Check sheet for the modelled part. Datum: model origin and axes. Units: mm. Give positions to 0.01 mm unless a question says otherwise; leave off trailing zeros. Order: outer loops, then holes, each group sorted by start corner. A loop starts at its lowest first (then second) coordinate and runs counter-clockwise, first axis right, second up.
from build123d import *

# Parameters (mm, degrees)
SKETCH1_W           = 85
SKETCH1_H           = 155
BOSS_EXTRUDE1_DEPTH = 20
SKETCH3_R           = 5.05
CUT_EXTRUDE1_DEPTH  = 10
SKETCH5_W           = 15
SKETCH5_H           = 50
BOSS_EXTRUDE2_DEPTH = 5
SKETCH6_R           = 3
CUT_EXTRUDE2_DEPTH  = 5


with BuildPart() as part:
    # Sketch1 → Boss-Extrude1 (new body)
    with BuildSketch(Plane(origin=(0, 0, 0), x_dir=(1, 0, 0), z_dir=(0, 1, 0))):
        with Locations((42.5, 77.5)):
            Rectangle(SKETCH1_W, SKETCH1_H)
    extrude(amount=BOSS_EXTRUDE1_DEPTH)

    # Sketch3 → Cut-Extrude1 (cut)
    with BuildSketch(Plane(origin=(0, 20, 0), x_dir=(1, 0, 0), z_dir=(0, 1, 0))):
        with Locations(Location((10, 145, 0), (0, 0, 270))):
            Circle(SKETCH3_R)
        with Locations(Location((25, 145, 0), (0, 0, 270))):
            Circle(SKETCH3_R)
        with Locations(Location((40, 145, 0), (0, 0, 270))):
            Circle(SKETCH3_R)
        with Locations(Location((55, 145, 0), (0, 0, 270))):
            Circle(SKETCH3_R)
        with Locations(Location((70, 145, 0), (0, 0, 270))):
            Circle(SKETCH3_R)
        with Locations(Location((70, 130, 0), (0, 0, 270))):
            Circle(SKETCH3_R)
        with Locations(Location((55, 130, 0), (0, 0, 270))):
            Circle(SKETCH3_R)
        with Locations(Location((40, 130, 0), (0, 0, 270))):
            Circle(SKETCH3_R)
        with Locations(Location((25, 130, 0), (0, 0, 270))):
            Circle(SKETCH3_R)
        with Locations(Location((10, 130, 0), (0, 0, 270))):
            Circle(SKETCH3_R)
        with Locations(Location((70, 115, 0), (0, 0, 270))):
            Circle(SKETCH3_R)
        with Locations(Location((55, 115, 0), (0, 0, 270))):
            Circle(SKETCH3_R)
        with Locations(Location((40, 115, 0), (0, 0, 270))):
            Circle(SKETCH3_R)
        with Locations(Location((25, 115, 0), (0, 0, 270))):
            Circle(SKETCH3_R)
        with Locations(Location((10, 115, 0), (0, 0, 270))):
            Circle(SKETCH3_R)
        with Locations(Location((70, 100, 0), (0, 0, 270))):
            Circle(SKETCH3_R)
        with Locations(Location((55, 100, 0), (0, 0, 270))):
            Circle(SKETCH3_R)
        with Locations(Location((40, 100, 0), (0, 0, 270))):
            Circle(SKETCH3_R)
        with Locations(Location((25, 100, 0), (0, 0, 270))):
            Circle(SKETCH3_R)
        with Locations(Location((10, 100, 0), (0, 0, 270))):
            Circle(SKETCH3_R)
        with Locations(Location((70, 85, 0), (0, 0, 270))):
            Circle(SKETCH3_R)
        with Locations(Location((55, 85, 0), (0, 0, 270))):
            Circle(SKETCH3_R)
        with Locations(Location((40, 85, 0), (0, 0, 270))):
            Circle(SKETCH3_R)
        with Locations(Location((25, 85, 0), (0, 0, 270))):
            Circle(SKETCH3_R)
        with Locations(Location((10, 85, 0), (0, 0, 270))):
            Circle(SKETCH3_R)
        with Locations(Location((70, 70, 0), (0, 0, 270))):
            Circle(SKETCH3_R)
        with Locations(Location((55, 70, 0), (0, 0, 270))):
            Circle(SKETCH3_R)
        with Locations(Location((40, 70, 0), (0, 0, 270))):
            Circle(SKETCH3_R)
        with Locations(Location((25, 70, 0), (0, 0, 270))):
            Circle(SKETCH3_R)
        with Locations(Location((10, 70, 0), (0, 0, 270))):
            Circle(SKETCH3_R)
        with Locations(Location((70, 55, 0), (0, 0, 270))):
            Circle(SKETCH3_R)
        with Locations(Location((55, 55, 0), (0, 0, 270))):
            Circle(SKETCH3_R)
        with Locations(Location((40, 55, 0), (0, 0, 270))):
            Circle(SKETCH3_R)
        with Locations(Location((25, 55, 0), (0, 0, 270))):
            Circle(SKETCH3_R)
        with Locations(Location((10, 55, 0), (0, 0, 270))):
            Circle(SKETCH3_R)
        with Locations(Location((70, 40, 0), (0, 0, 270))):
            Circle(SKETCH3_R)
        with Locations(Location((55, 40, 0), (0, 0, 270))):
            Circle(SKETCH3_R)
        with Locations(Location((40, 40, 0), (0, 0, 270))):
            Circle(SKETCH3_R)
        with Locations(Location((25, 40, 0), (0, 0, 270))):
            Circle(SKETCH3_R)
        with Locations(Location((10, 40, 0), (0, 0, 270))):
            Circle(SKETCH3_R)
        with Locations(Location((70, 25, 0), (0, 0, 270))):
            Circle(SKETCH3_R)
        with Locations(Location((55, 25, 0), (0, 0, 270))):
            Circle(SKETCH3_R)
        with Locations(Location((40, 25, 0), (0, 0, 270))):
            Circle(SKETCH3_R)
        with Locations(Location((25, 25, 0), (0, 0, 270))):
            Circle(SKETCH3_R)
        with Locations(Location((10, 25, 0), (0, 0, 270))):
            Circle(SKETCH3_R)
        with Locations(Location((70, 10, 0), (0, 0, 270))):
            Circle(SKETCH3_R)
        with Locations(Location((55, 10, 0), (0, 0, 270))):
            Circle(SKETCH3_R)
        with Locations(Location((40, 10, 0), (0, 0, 270))):
            Circle(SKETCH3_R)
        with Locations(Location((25, 10, 0), (0, 0, 270))):
            Circle(SKETCH3_R)
        with Locations(Location((10, 10, 0), (0, 0, 270))):
            Circle(SKETCH3_R)
    extrude(amount=-CUT_EXTRUDE1_DEPTH, mode=Mode.SUBTRACT)

    # Sketch5 → Boss-Extrude2 (add)
    with BuildSketch(Plane(origin=(85, 0, 0), x_dir=(0, 0, -1), z_dir=(1, 0, 0))):
        with Locations((17.5, 10)):
            Rectangle(SKETCH5_W, SKETCH5_H)
        with Locations((137.5, 10)):
            Rectangle(SKETCH5_W, SKETCH5_H)
    extrude(amount=BOSS_EXTRUDE2_DEPTH)

    # Sketch6 → Cut-Extrude2 (cut)
    with BuildSketch(Plane(origin=(90, 0, 0), x_dir=(0, 0, -1), z_dir=(1, 0, 0))):
        with Locations((17.5, 27.5)):
            Circle(SKETCH6_R)
        with Locations((17.5, -7.5)):
            Circle(SKETCH6_R)
        with Locations((137.5, -7.5)):
            Circle(SKETCH6_R)
        with Locations((137.5, 27.5)):
            Circle(SKETCH6_R)
    extrude(amount=-CUT_EXTRUDE2_DEPTH, mode=Mode.SUBTRACT)


solid = part.part
1) Section check A-A, the plane y = 22. Record the cut outline in (x, z).
Recorded:
outline: (85, -145) - (90, -145) - (90, -130) - (85, -130) - close; (85, -25) - (90, -25) - (90, -10) - (85, -10) - close
2) Section check D-D, the plane x = 81.5. Record the cut outline in (y, z), then the cut area to 3 significant figures.
Recorded:
outline: (0, -155) - (20, -155) - (20, 0) - (0, 0) - close
area: 3,100 mm2
3) Material ranges on L1, parallel to X at y = 17.5, z = -40; L2, parallel to Y at x = 88.8, z = -137.5; L3, parallel to Z at x = 87, y = 27, recorded low to high.
Recorded:
L1: x = 0 to 4.95, 15.05 to 19.95, 30.05 to 34.95, 45.05 to 49.95, 60.05 to 64.95, 75.05 to 85
L2: y = -15 to -10.5, -4.5 to 24.5, 30.5 to 35
L3: z = -145 to -140.46, -134.54 to -130, -25 to -20.46, -14.54 to -10
4) Section check B-B, the plane y = -7.5. Record the cut outline in (x, z).
Recorded:
outline: (85, -145) - (90, -145) - (90, -140.5) - (85, -140.5) - close; (85, -134.5) - (90, -134.5) - (90, -130) - (85, -130) - close; (85, -25) - (90, -25) - (90, -20.5) - (85, -20.5) - close; (85, -14.5) - (90, -14.5) - (90, -10) - (85, -10) - close
5) Draft check along X on faces 1 (the face through (25, 10, -70)), 2 (the face through (87.5, 25.7, -15.1)), 3 (the face through (90, 10, -17)). Enter one of: +X half, -X half, draft (parallel to the pull), parting line (faces both ways), or undercut.
Recorded:
face 1: undercut
face 2: draft
face 3: +X half
6) Depth check by flat-ended pin: pin 1 Ø11 at (x, z) = (11.5, -85.5) entering from +Y; pin 2 Ø9 at (x, z) = (10, -145) entering from -Y; pin 3 Ø4 at (y, z) = (-8, -134) entering from -X. Enter the tip coordinate at first touch or a pass-through.
Recorded:
pin 1: stops at y = 20
pin 2: stops at y = 0
pin 3: stops at x = 85
7) Section check C-C, the plane z = -40. Record the cut outline in (x, y), then the cut area to 4 significant figures.
Recorded:
outline: (0, 0) - (85, 0) - (85, 20) - (75.05, 20) - (75.05, 10) - (64.95, 10) - (64.95, 20) - (60.05, 20) - (60.05, 10) - (49.95, 10) - (49.95, 20) - (45.05, 20) - (45.05, 10) - (34.95, 10) - (34.95, 20) - (30.05, 20) - (30.05, 10) - (19.95, 10) - (19.95, 20) - (15.05, 20) - (15.05, 10) - (4.95, 10) - (4.95, 20) - (0, 20) - close
area: 1,195 mm2
